Geometry: see drawing. Coordinates: mm, zero at the bounding-box minimum. Round coordinates to 2 decimals unless told otherwise and drop trailing zeros. Loops run counter-clockwise (first coordinate to the right, second up) from the corner with the lowest first, then second, coordinate; pieces in that order, holes last.
(1) Section B-B, the plane y = 3.65. Return the cut outline in (x, z) (1 decimal).
(2) Material intervals for probe 1 along Y at (x, z) = (48, 3); probe 2 along Z at (x, y) = (55, 3.95) (1 decimal); probe 3 along Z at (x, y) = (19, 2.1) (1 decimal), sorted ascending.
(3) Section C-C, the plane z = 3. Return the cut outline in (x, y).
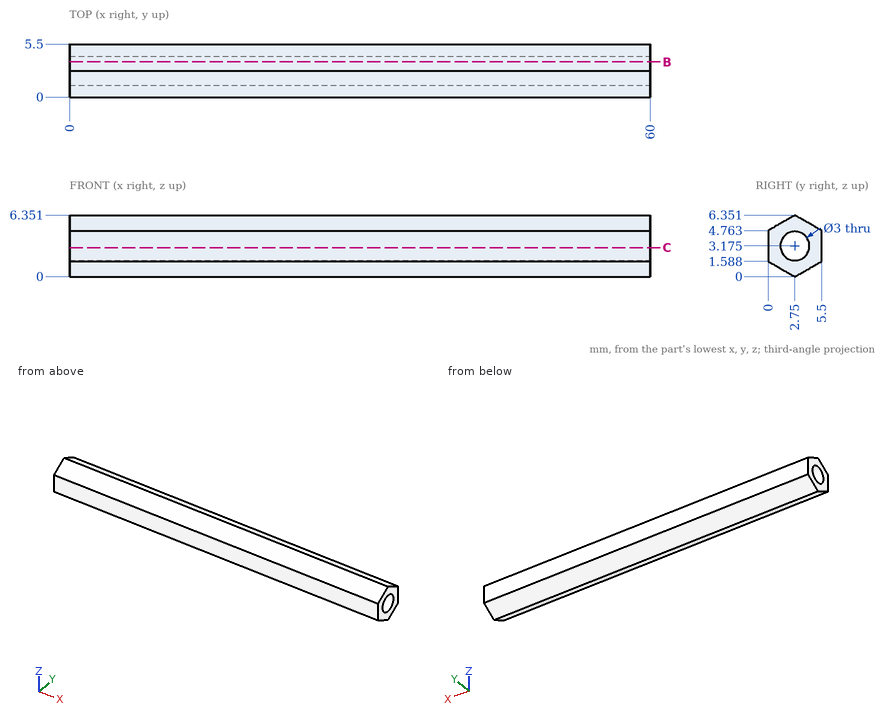
Output values:
1. outline: (0, 0.5) - (60, 0.5) - (60, 2) - (0, 2) - close; (0, 4.4) - (60, 4.4) - (60, 5.8) - (0, 5.8) - close
2. probe 1: y = 0 to 1.26, 4.24 to 5.5
2. probe 2: z = 0.7 to 2.3, 4.1 to 5.7
2. probe 3: z = 0.4 to 1.8, 4.5 to 6
3. outline: (0, 0) - (60, 0) - (60, 1.26) - (0, 1.26) - close; (0, 4.24) - (60, 4.24) - (60, 5.5) - (0, 5.5) - close
